Geometry check sheet. Reference: the model listing, model coordinates, mm. A direction names the side the tool comes from. Coordinates: 2 decimals unless noted, no trailing zeros. Write each loop counter-clockwise with the first axis right and the second up, starting at its lowest first coordinate (ties: lowest second). Pieces come first, ordered by that corner, then holes. Notation, with made-up numbers: (2, 56.25) -> (31, 56.25) arc R37 ccw to (31, 92.25) -> close; hole circle Ø5 at (68.25, 50). An arc over 180 degrees is marked (long way). One line per question, with ' | ' between items.
```python
from build123d import *

# Parameters (mm, degrees)
SKETCH1_R           = 4
BOSS_EXTRUDE1_DEPTH = 7
BOSS_EXTRUDE2_START = 7
SKETCH1_4_R         = 4
BOSS_EXTRUDE2_DEPTH = 7


with BuildPart() as part:
    # Sketch1 → Boss-Extrude1 (new body)
    # profile 1 of 2: a face of its own
    with BuildSketch(Plane(origin=(0, 0, 0), x_dir=(0, 0, -1), z_dir=(1, 0, 0))):
        Polygon((-10, 6), (-10, -6), (-5, -11), (9.5, -11), (9.5, -9), (70, -9), (70, 11), (-5, 11), align=None)
        Circle(SKETCH1_R, mode=Mode.SUBTRACT)
        with BuildLine():
            ThreePointArc((63, 6.75), (61.25, 5), (63, 3.25))
            Line((63, 3.25), (65, 3.25))
            ThreePointArc((65, 3.25), (66.75, 5), (65, 6.75))
            Line((65, 6.75), (63, 6.75))
        make_face(mode=Mode.SUBTRACT)
        with BuildLine():
            ThreePointArc((46, -6.75), (47.75, -5), (46, -3.25))
            Line((46, -3.25), (44, -3.25))
            ThreePointArc((44, -3.25), (42.25, -5), (44, -6.75))
            Line((44, -6.75), (46, -6.75))
        make_face(mode=Mode.SUBTRACT)
        with BuildLine():
            ThreePointArc((27, 3.25), (28.75, 5), (27, 6.75))
            Line((27, 6.75), (25, 6.75))
            ThreePointArc((25, 6.75), (23.25, 5), (25, 3.25))
            Line((25, 3.25), (27, 3.25))
        make_face(mode=Mode.SUBTRACT)
    # profile 2 of 2: a face of its own
    with BuildSketch(Plane(origin=(0, 0, 0), x_dir=(0, 0, -1), z_dir=(1, 0, 0))):
        Circle(SKETCH1_R)
    extrude(amount=BOSS_EXTRUDE1_DEPTH)

    # Sketch1<4> → Boss-Extrude2 (add)
    with BuildSketch(Plane(origin=(0, 0, 0), x_dir=(0, 0, -1), z_dir=(1, 0, 0)).offset(BOSS_EXTRUDE2_START)):
        Circle(SKETCH1_4_R)
    extrude(amount=BOSS_EXTRUDE2_DEPTH)


solid = part.part
```
(1) Draft check along Y on faces 1 (the face through (0, 0, -29)), 2 (the face through (3, 11, -33)), 3 (the face through (3, 3.25, -26)). Enter one of: pulls with the +Y half, pulls with the -Y half, needs draft (parallel to the pull), parting line crosses it, or undercut.
Answers below:
face 1: needs draft | face 2: pulls with the +Y half | face 3: undercut
(2) Tool access check on faces 4 (the face through (3, 0, 10)), 5 (the face through (3, -3.25, -45)), 6 (the face through (3, -10, -9.5)). Record the directions out of +Z, -Z, +X, -X, +Y, -Y that give a thin tool (end or side, any length) a straight path to the whole face; none if there is none.
Answers below:
face 4: +Z, +X, -X, +Y, -Y | face 5: +X, -X | face 6: -Z, +X, -X, -Y
(3) Cross-section at D-D (z = 0). Record the cut outline in (x, y), plus the area to 3 significant figures.
Answers below:
outline: (0, -11) -> (7, -11) -> (7, -4) -> (14, -4) -> (14, 4) -> (7, 4) -> (7, 11) -> (0, 11) -> close | area: 210 mm²
(4) Cross-section at C-C (y = 0). Record the cut outline in (x, z).
Answers below:
outline: (0, -70) -> (7, -70) -> (7, -4) -> (14, -4) -> (14, 4) -> (7, 4) -> (7, 10) -> (0, 10) -> close
(5) Cross-section at A-A (x = 2.75). Record the cut outline in (y, z), plus the area to 3 significant figures.
Answers below:
outline: (-11, -9.5) -> (-9, -9.5) -> (-9, -70) -> (11, -70) -> (11, 5) -> (6, 10) -> (-6, 10) -> (-11, 5) -> close; hole (-6.75, -46) arc R1.75 ccw to (-3.25, -46) -> (-3.25, -44) arc R1.75 ccw to (-6.75, -44) -> close; hole (3.25, -65) arc R1.75 ccw to (6.75, -65) -> (6.75, -63) arc R1.75 ccw to (3.25, -63) -> close; hole (3.25, -27) arc R1.75 ccw to (6.75, -27) -> (6.75, -25) arc R1.75 ccw to (3.25, -25) -> close | area: 1,560 mm²
(6) Depth check by flat-ended pin: P1, Ø1, axis at x = 4, y = -10.5, coming from the -Z side; P2, Ø2, axis at x = 3, z = -26, coming from the -Y side; P3, Ø6.5, axis at y = 5, z = -11.5, coming from the +X side. Enter the tip coordinate at first touch or a pass-through.
Answers below:
P1: stops at z = -9.5 | P2: stops at y = -9 | P3: stops at x = 7
(7) Cross-section at B-B (y = -5). Record the cut outline in (x, z).
Answers below:
outline: (0, -70) -> (7, -70) -> (7, -47.75) -> (0, -47.75) -> close; (0, -42.25) -> (7, -42.25) -> (7, 10) -> (0, 10) -> close
(8) Material ranges on line 1 (Z direction, x = 4, y = 4.5); line 2 (X direction, y = -2.25, z = -4.5); line 3 (Y direction, x = 4.75, z = -65), recorded low to high.
Answers below:
line 1: z = -70 to -66.68, -61.32 to -28.68, -23.32 to 10 | line 2: x = 0 to 7 | line 3: y = -9 to 3.25, 6.75 to 11
